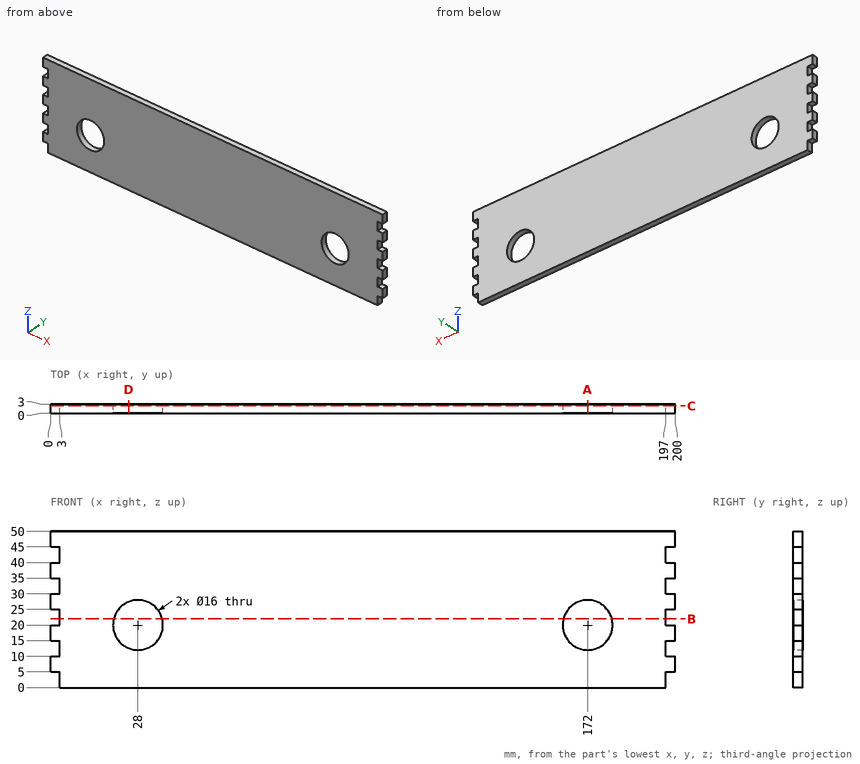
Source: three-view drawing plus pictorial views. Frame: mm from the lowest corner of the part. Give positions to 0.01 mm unless a question says otherwise; leave off trailing zeros. Order: outer loops, then holes, each group sorted by start corner. A loop starts at its lowest first (then second) coordinate and runs counter-clockwise, first axis right, second up. Notation, with made-up numbers: (35.25, -38) - (77.25, -38) arc R11 cw to (77.25, -33) - close; hole circle Ø11 at (29, 18.25). An arc over 180 degrees is marked (long way). Put each result on its own line as item: value.
Item 1: Ray query, L1, parallel to Z at x = 28, y = 1.55; L2, parallel to X at y = 2.6, z = 14; L3, parallel to X at y = 2.7, z = 24.5. Return the intervals inside material, ascending. Write a range as from..to.
Found:
L1: z = 0..12, 28..50
L2: x = 3..22.71, 33.29..166.71, 177.29..197
L3: x = 3..21.39, 34.61..165.39, 178.61..197
Item 2: Section query C-C, the plane y = 2.4. Count the separate pieces of the cut face and the enclosed holes in it, then the cut area to 3 significant figures.
Found:
separate pieces: 1
enclosed holes: 2
area: 9,450 mm^2
Item 3: Section query B-B, the plane z = 22. Return loops of the section in (x, y), then the cut area to 3 significant figures.
Found:
outline: (3, 0) - (20.25, 0) - (20.25, 3) - (3, 3) - close; (35.75, 0) - (164.25, 0) - (164.25, 3) - (35.75, 3) - close; (179.75, 0) - (197, 0) - (197, 3) - (179.75, 3) - close
area: 489 mm^2
Item 4: Section query D-D, the plane x = 25. Return loops of the section in (y, z), then the cut area to 3 significant figures.
Found:
outline: (0, 0) - (3, 0) - (3, 12.58) - (0, 12.58) - close; (0, 27.42) - (3, 27.42) - (3, 50) - (0, 50) - close
area: 106 mm^2
Item 5: Contact query for flat-ended pins moving along their axis: pin 1 (1 mm diameter, centred on x = 104, z = 41, fed in from -Y); pin 2 (0.9 mm diameter, centred on x = 1.5, y = 1.5, fed in from -Z); pin 3 (1 mm diameter, centred on y = 2, z = 41.5, fed in from -X). Output: stop coordinate, or through.
Found:
pin 1: stops at y = 0
pin 2: stops at z = 5
pin 3: stops at x = 3
Item 6: Section query A-A, the plane x = 172. Return loops of the section in (y, z), then the cut area to 3 significant figures.
Found:
outline: (0, 0) - (3, 0) - (3, 12) - (0, 12) - close; (0, 28) - (3, 28) - (3, 50) - (0, 50) - close
area: 102 mm^2
